Verification items for the finished model (mm, model axes). A direction names the side the tool comes from. Give positions to 0.01 mm unless a question says otherwise; leave off trailing zeros. Order: outer loops, then holes, each group sorted by start corner. A loop starts at its lowest first (then second) coordinate and runs counter-clockwise, first axis right, second up.
from build123d import *

# Parameters (mm, degrees)
F1_DEPTH = 25.4
F2_DEPTH = 101.6
F3_W     = 127
F3_H     = 50.8
F5_DEPTH = 25.4


with BuildPart() as f1:
    # F0 (on Front) → F1 (new body)
    with BuildSketch(Plane.XZ):
        Polygon((-6.504758, -12.474676), (-31.904758, -12.474676), (-31.904758, -37.874676), (31.595242, -37.874676), (31.595242, 38.325324), (-6.504758, 38.325324), align=None)
    extrude(amount=F1_DEPTH)

    # F1_face (on face) → F2 (join)
    with BuildSketch(Plane(origin=(6.772515, -25.4, -4.392858), x_dir=(1, 0, 0), z_dir=(0, -1, 0))):
        Polygon((-13.277273, 42.718182), (-13.277273, -8.081818), (-38.677273, -8.081818), (-38.677273, -33.481818), (24.822727, -33.481818), (24.822727, 42.718182), align=None)
    extrude(amount=F2_DEPTH)

    # F3 (on face) → F5 (cut)
    with BuildSketch(Plane(origin=(-6.504758, 0, 0), x_dir=(0, -1, 0), z_dir=(-1, 0, 0))):
        with Locations((63.5, 12.925324)):
            Rectangle(F3_W, F3_H)
    extrude(amount=-F5_DEPTH, mode=Mode.SUBTRACT)


solid = f1.part
(1) Go/stop test with a flat-tipped pin: pin 1 (15 mm diameter, centred on x = -9, y = -64, fed in from +Z). Record where the tip stops, or that it passes through.
Solved:
pin 1: stops at z = -12.47
(2) Section check A-A, the plane x = -27. Enter the section's corners in (y, z), then the cut area to 3 significant figures.
Solved:
outline: (-127, -37.87) - (0, -37.87) - (0, -12.47) - (-127, -12.47) - close
area: 3,230 mm2
(3) Section check C-C, the plane z = 14.5. Enter the section's corners in (x, y).
Solved:
outline: (18.9, -127) - (31.6, -127) - (31.6, 0) - (18.9, 0) - close
(4) Set-up check for faces 1 (the flat face through (-6, -63, -12.475)), 2 (the flat face through (-31.905, -63, -25)): record each of +Z, -Z, +X, -X, +Y, -Y from which the full face is reachable in a straight line by a thin tool's end or side.
Solved:
face 1: +Z, -X, +Y, -Y
face 2: +Z, -Z, -X, +Y, -Y
(5) Scan lines: line 1 (Z direction, x = -22, y = -61); line 2 (X direction, y = -70, z = 29). Record each from-to range of solid material in increasing order.
Solved:
line 1: z = -37.87 to -12.47
line 2: x = 18.9 to 31.6
(6) Section check B-B, the plane y = -94.5. Enter the section's corners in (x, z), then the cut area to 3 significant figures.
Solved:
outline: (-31.9, -37.87) - (31.6, -37.87) - (31.6, 38.33) - (18.9, 38.33) - (18.9, -12.47) - (-31.9, -12.47) - close
area: 2,260 mm2
